Can you work these out from the drawing? Everything is in mm from the part's minimum corner. A direction names the side the tool comes from. Round coordinates to 2 decimals unless told otherwise and drop trailing zeros. Write each loop counter-clockwise with the first axis right and the second up, starting at its lowest first coordinate (ties: lowest second). Pieces come first, ordered by that corner, then holes. Notation, with made-up numbers: (-25, 24) - (3, 24) arc R20 ccw to (3, 46) - close; hole circle Ø5 at (23, -30). An arc over 180 degrees is marked (long way). Write each question's results on one line, items separated by ' | '. Start each with the question number.
(1) Imagine slicing it at A-A on z = 3. Write out the boundary of the cut face in (x, y).
(2) For P1, Ø2, axis at x = 15, y = 1, coming from the -Z side; P2, Ø1.5, axis at x = 11, z = 4, coming from the +Y side, each with a flat end and sliding along its axis, tell me the tip position at first contact or that it passes through.
(3) Please list where these lines run through material, in increasing order: line 1 (X direction, y = 1, z = 5.1); line 2 (Z direction, x = 14.5, y = 5.75); line 3 (Z direction, x = 12.5, y = 3.15). Write a range as [from, to].
(4) Imagine slicing it at C-C on x = 4.5. Write out the boundary of the cut face in (y, z).
(5) Imagine slicing it at B-B on y = 3. Write out the boundary of the cut face in (x, z), then the cut area to 3 significant figures.
(6) On a 3-axis mill with a long thin cutter (end or side, diameter ignored), from which of +Z, -Z, +X, -X, +Y, -Y can I reach the whole of each face in a straight line? I mean the marked faces 1 and 2. Say none if no direction works.
(7) Imagine slicing it at D-D on z = 1. Write out the boundary of the cut face in (x, y).
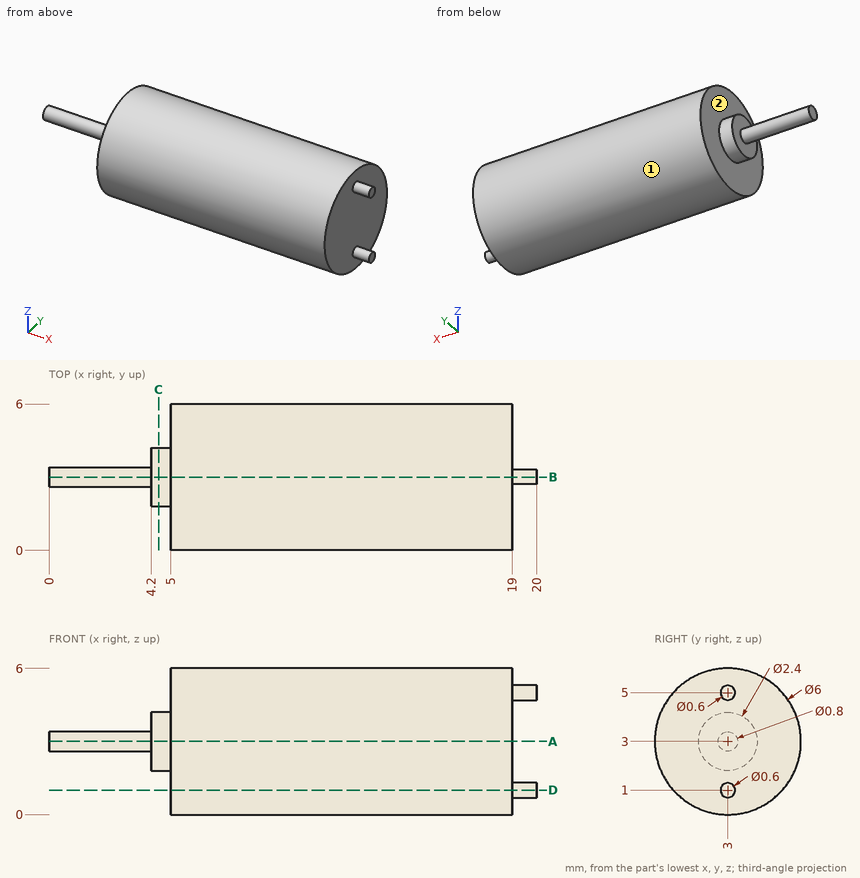
Response:
1) outline: (0, 2.6) - (4.2, 2.6) - (4.2, 1.8) - (5, 1.8) - (5, 0) - (19, 0) - (19, 6) - (5, 6) - (5, 4.2) - (4.2, 4.2) - (4.2, 3.4) - (0, 3.4) - close
2) P1: z = 0.17 | P2: y = 5.99
3) line 1: [5, 19] | line 2: [1.8, 4.2] | line 3: [0, 6]
4) outline: circle Ø2.4 at (3, 3)
5) outline: (0, 2.6) - (4.2, 2.6) - (4.2, 1.8) - (5, 1.8) - (5, 0) - (19, 0) - (19, 0.7) - (20, 0.7) - (20, 1.3) - (19, 1.3) - (19, 4.7) - (20, 4.7) - (20, 5.3) - (19, 5.3) - (19, 6) - (5, 6) - (5, 4.2) - (4.2, 4.2) - (4.2, 3.4) - (0, 3.4) - close | area: 90.5 mm²
6) face 1: +X, -X | face 2: -X
7) outline: (5, 0.76) - (19, 0.76) - (19, 2.7) - (20, 2.7) - (20, 3.3) - (19, 3.3) - (19, 5.24) - (5, 5.24) - close
